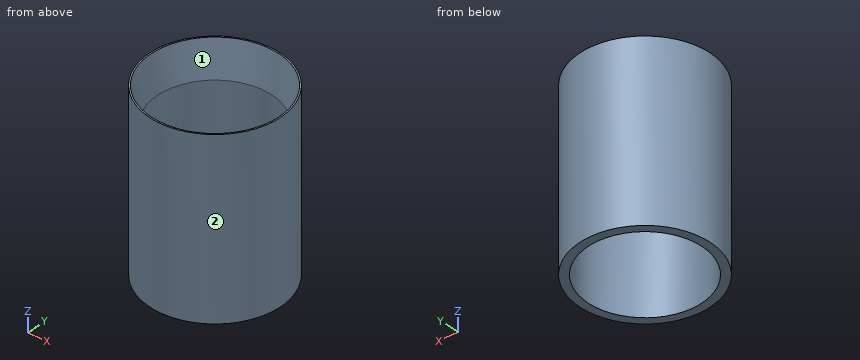
from build123d import *

# Parameters (mm, degrees)
F0_R     = 9.525
F1_DEPTH = 25.4
F2_T     = -1.2
F3_SIZE2 = 0.9966563757
F3_SIZE  = 5.08


with BuildPart() as f1:
    # F0 (on Top) → F1 (new body)
    with BuildSketch(Plane.XY):
        Circle(F0_R)
    extrude(amount=F1_DEPTH)

    # F2
    f2_openings = [f1.faces().sort_by_distance(p)[0] for p in [
        (0, 0, 25.4),
        (0, 0, 0),
    ]]
    offset(amount=F2_T, openings=f2_openings)

    # F3
    f3_edges = [f1.edges().sort_by_distance(p)[0] for p in [
        (-8.325, 0, 25.4),
    ]]
    chamfer(f3_edges, length=F3_SIZE, length2=F3_SIZE2)


solid = f1.part
Input: part model. Units: mm. Frame: model coordinates. Face numbers are marked on the shaded views. Round coordinates to 2 decimals unless told otherwise and drop trailing zeros. Order: outer loops, then holes, each group sorted by start corner. A loop starts at its lowest first (then second) coordinate and runs counter-clockwise, first axis right, second up. Notation, with made-up numbers: (38, 74.25) - (51, 74.25) arc R7 ccw to (51, 86.25) - close; hole circle Ø7 at (-37.75, 74). An arc over 180 degrees is marked (long way). Use a Markdown table: item, result.
1. Section C-C on z = 1.5. Return the cut outline in (x, y) (3 decimals).
Evaluation:
| item | result |
|---|---|
| outline | circle Ø19.05 at (0, 0); hole circle Ø16.65 at (0, 0) |
2. Mould query, pull axis X, two halves, no side actions, for the marked faces 1 and 2. Classes: +X half, -X half, draft (parallel to the pull), parting line (faces both ways), or undercut.
Evaluation:
| item | result |
|---|---|
| face 1 | undercut |
| face 2 | parting line |
3. Material intervals for probe 1 along Y at (x, z) = (0, 6.25) (3 decimals); probe 2 along Y at (x, z) = (-3, 18); probe 3 along X at (y, z) = (-7, 24.25), sorted ascending.
Evaluation:
| item | result |
|---|---|
| probe 1 | -9.525 to -8.325, 8.325 to 9.525 |
| probe 2 | -9.04 to -7.77, 7.77 to 9.04 |
| probe 3 | -6.46 to -5.81, 5.81 to 6.46 |
4. Section A-A on y = 0. Return the cut outline in (x, z) (3 decimals), then the cut area to 3 significant figures.
Evaluation:
| item | result |
|---|---|
| outline | (-9.525, 0) - (-8.325, 0) - (-8.325, 20.32) - (-9.322, 25.4) - (-9.525, 25.4) - close; (8.325, 0) - (9.525, 0) - (9.525, 25.4) - (9.322, 25.4) - (8.325, 20.32) - close |
| area | 55.9 mm^2 |
5. First-contact query: pin 1 (10 mm diameter, centred on x = -6.5, z = 15, fed in from -Y); pin 2 (3 mm diameter, centred on y = -2, z = 4.5, fed in from +X); pin 3 (3 mm diameter, centred on y = -3, z = 8.5, fed in from -X). Flat tips, straight axial feed; report the tip coordinate or a pass-through.
Evaluation:
| item | result |
|---|---|
| pin 1 | y = -9.41 |
| pin 2 | x = 9.51 |
| pin 3 | x = -9.41 |
6. Section D-D on z = 23. Return the cut outline in (x, y) (3 decimals).
Evaluation:
| item | result |
|---|---|
| outline | circle Ø19.05 at (0, 0); hole circle Ø17.702 at (0, 0) |
